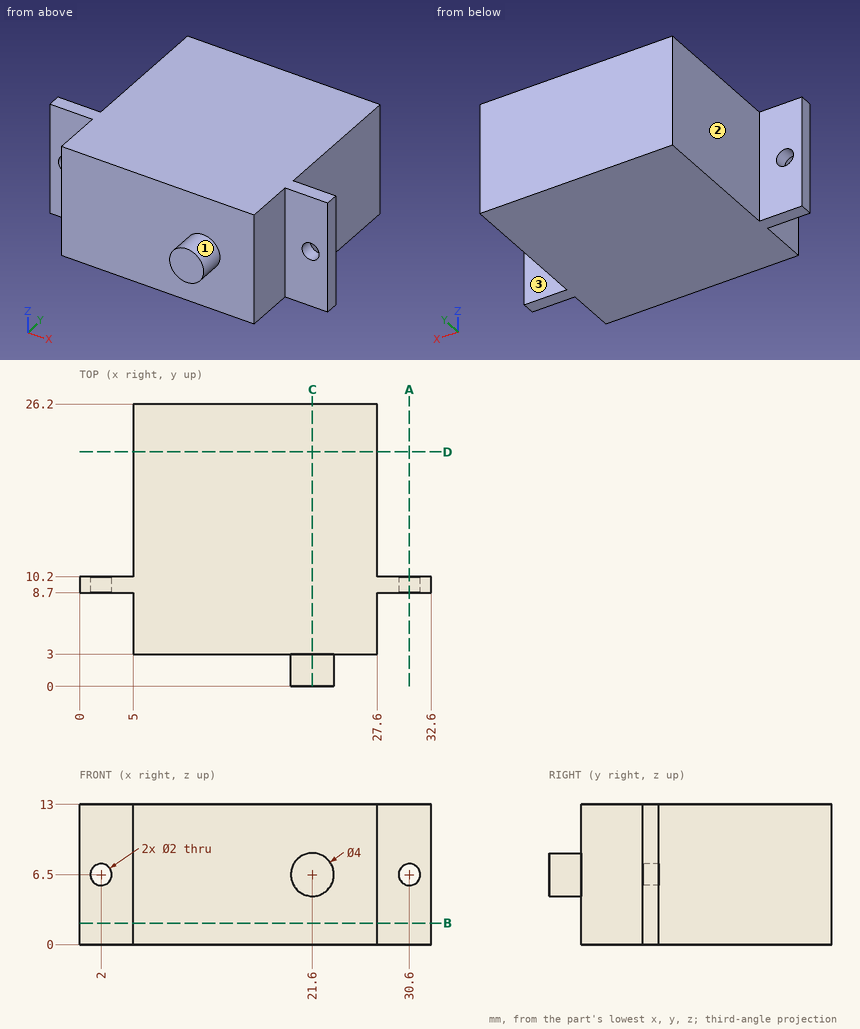
Drawing for the job (mm, zero at the part's lowest x, y, z). A direction names the side the tool comes from. Coordinates: 2 decimals unless noted, no trailing zeros. Order: outer loops, then holes, each group sorted by start corner. A loop starts at its lowest first (then second) coordinate and runs counter-clockwise, first axis right, second up. Notation, with made-up numbers: (32, 4) -> (39, 4) arc R21 cw to (39, 15) -> close; hole circle Ø5 at (-6, 22). An arc over 180 degrees is marked (long way). Answer in a Markdown table with one row per item.
1) Flat gauge pins, fed straight in: P1, Ø2.5, axis at x = 2, z = 6.5, coming from the -Y side; P2, Ø5.5, axis at x = 30, z = 9, coming from the -Y side; P3, Ø6.5, axis at y = 17.5, z = 9, coming from the +X side. Where does each tip first touch, or does it go through?
Check values:
| item | result |
|---|---|
| P1 | y = 8.7 |
| P2 | y = 3 |
| P3 | x = 27.6 |
2) Drill centre lines: line 1 (Z direction, x = 2, y = 9.2); line 2 (Y direction, x = 3.5, z = 2.5); line 3 (X direction, y = 4.5, z = 11.25). Where is each one in solid material? Low to high.
Check values:
| item | result |
|---|---|
| line 1 | 0 to 5.5, 7.5 to 13 |
| line 2 | 8.7 to 10.2 |
| line 3 | 5 to 27.6 |
3) Band-saw the part on D-D (y = 21.75). List the corners of the cut face in (x, z).
Check values:
| item | result |
|---|---|
| outline | (5, 0) -> (27.6, 0) -> (27.6, 13) -> (5, 13) -> close |
4) Band-saw the part on A-A (x = 30.6). List the corners of the cut face in (y, z), and give its area (3 significant figures).
Check values:
| item | result |
|---|---|
| outline | (8.7, 0) -> (10.2, 0) -> (10.2, 5.5) -> (8.7, 5.5) -> close; (8.7, 7.5) -> (10.2, 7.5) -> (10.2, 13) -> (8.7, 13) -> close |
| area | 16.5 mm2 |
5) Band-saw the part on B-B (z = 2). List the corners of the cut face in (x, y), and give its area (3 significant figures).
Check values:
| item | result |
|---|---|
| outline | (0, 8.7) -> (5, 8.7) -> (5, 3) -> (27.6, 3) -> (27.6, 8.7) -> (32.6, 8.7) -> (32.6, 10.2) -> (27.6, 10.2) -> (27.6, 26.2) -> (5, 26.2) -> (5, 10.2) -> (0, 10.2) -> close |
| area | 539 mm2 |
6) Band-saw the part on C-C (x = 21.6). List the corners of the cut face in (y, z), and give its area (3 significant figures).
Check values:
| item | result |
|---|---|
| outline | (0, 4.5) -> (3, 4.5) -> (3, 0) -> (26.2, 0) -> (26.2, 13) -> (3, 13) -> (3, 8.5) -> (0, 8.5) -> close |
| area | 314 mm2 |
7) Which spindle directions (+Z, -Z, +X, -X, +Y, -Y) get a long thin tool onto all of the face, cutting with end or side? Do the marked faces 1, 2 and 3. Say none if no direction does.
Check values:
| item | result |
|---|---|
| face 1 | -Y |
| face 2 | +Z, -Z, -X, +Y |
| face 3 | +Z, -Z, +X, +Y |
